```python
from build123d import *

# Parameters (mm, degrees)
F0_W     = 72
F0_H     = 24
F1_DEPTH = 27
F2_T     = -1
F3_R     = 3.25
F4_DEPTH = 25
F5_W     = 72
F5_H     = 27
F5_R     = 3.25
F6_DEPTH = 1
F8_DEPTH = 1
F9_R     = 0.8


# Not quite as in the source:
# - a feature names something its author has since deleted; it is built from what else it names


with BuildPart() as f1:
    # F0 (on Front) → F1 (new body)
    with BuildSketch(Plane.XZ):
        Rectangle(F0_W, F0_H)
    extrude(amount=F1_DEPTH)

    # F2
    f2_openings = [f1.faces().sort_by_distance(p)[0] for p in [
        (36, -13.5, 0),
    ]]
    offset(amount=F2_T, openings=f2_openings)

    # F3 (on face) → F4 (cut)
    with BuildSketch(Plane.XY.offset(12)):
        with Locations((-18.75, -13.5)):
            Circle(F3_R)
    extrude(amount=-F4_DEPTH, mode=Mode.SUBTRACT)

    # F5 (on face) → F6 (cut)
    with BuildSketch(Plane(origin=(0, 0, -12), x_dir=(1, 0, 0), z_dir=(0, 0, -1))):
        with Locations((0, 13.5)):
            Rectangle(F5_W, F5_H)
        with Locations((-18.75, 13.5)):
            Circle(F5_R, mode=Mode.SUBTRACT)
    extrude(amount=-F6_DEPTH, mode=Mode.SUBTRACT)

    # F9
    f9_edges = [f1.edges().sort_by_distance(p)[0] for p in [
        (-36, -27, 0.5),
        (-36, 0, 0.5),
    ]]
    fillet(f9_edges, radius=F9_R)


with BuildPart() as f8:
    # F7 (on face) → F8 (new body)
    with BuildSketch(Plane.XY.offset(12)):
        with BuildLine():
            Line((-36, -1), (-36, -27))
            Line((-36, -27), (36, -27))
            Line((36, -27), (36, -16.75))
            Line((36, -16.75), (-18.75, -16.75))
            ThreePointArc((-18.75, -16.75), (-22, -13.5), (-18.75, -10.25))
            Line((-18.75, -10.25), (36, -10.25))
            Line((36, -10.25), (36, -1))
            Line((36, -1), (-36, -1))
        make_face()
    extrude(amount=F8_DEPTH)


solid = f1.part
```
Build history of the part. All positions in model axes, mm. A direction names the side the tool comes from. Round coordinates to 2 decimals unless told otherwise and drop trailing zeros. Write each loop counter-clockwise with the first axis right and the second up, starting at its lowest first coordinate (ties: lowest second). Pieces come first, ordered by that corner, then holes.
1) Band-saw the part on B-B, the plane x = -18.75. List the corners of the cut face in (y, z).
2) Mould opens along Y. For faces 3 (the flat face through (0, 0, 1)), 4 (the flat face through (-36, -13, 0)), 5 (the cylindrical face through (-22, -13.4, 11.5)), 6 (the flat face through (0, -13, 11)) say: +Y half, -Y half, draft (parallel to the pull), parting line (faces both ways), or undercut.
3) Drill centre lines: probe 1 along Y at (x, z) = (-33, 5); probe 2 along Y at (x, z) = (-18.75, 11.6); probe 3 along Z at (x, y) = (31.5, -8.75). Where is each one in solid material? Low to high.
4) Band-saw the part on D-D, the plane z = -3. List the corners of the cut face in (x, y).
5) Pin check, flat tips, straight feed: pin 1 (1 mm diameter, centred on y = -5.5, z = 0, fed in from +X); pin 2 (2 mm diameter, centred on x = 12.5, y = -19.5, fed in from -Z). Stop position of each tip, or through.
6) Band-saw the part on A-A, the plane y = -13.5. List the corners of the cut face in (x, z), and give its area (3 significant figures).
7) Band-saw the part on C-C, the plane x = -26.5. List the corners of the cut face in (y, z).
8) 3-axis set-ups, long thin cutter, end or side, ignore diameter. For faces 1 (the flat face through (-0.2, -0.6, -11)), 2 (the flat face through (-35, -13, 0)): which of +Z, -Z, +X, -X, +Y, -Y reach the whole face in a straight line?
Ans:
1. outline: (-27, -11) - (-26, -11) - (-26, 11) - (-16.75, 11) - (-16.75, 12) - (-27, 12) - close; (-10.25, 11) - (-1, 11) - (-1, -11) - (0, -11) - (0, 12) - (-10.25, 12) - close
2. face 3: +Y half
2. face 4: draft
2. face 5: undercut
2. face 6: undercut
3. probe 1: y = -27 to -26, -1 to 0
3. probe 2: y = -27 to -16.75, -10.25 to 0
3. probe 3: z = 11 to 12
4. outline: (-36, -26.2) arc R0.8 ccw to (-35.2, -27) - (36, -27) - (36, -26) - (-35, -26) - (-35, -1) - (36, -1) - (36, 0) - (-35.2, 0) arc R0.8 ccw to (-36, -0.8) - close
5. pin 1: stops at x = -35
5. pin 2: stops at z = 11
6. outline: (-36, -11) - (-35, -11) - (-35, 11) - (-22, 11) - (-22, 12) - (-36, 12) - close; (-15.5, 11) - (36, 11) - (36, 12) - (-15.5, 12) - close
6. area: 87.5 mm2
7. outline: (-27, -11) - (-26, -11) - (-26, 11) - (-1, 11) - (-1, -11) - (0, -11) - (0, 12) - (-27, 12) - close
8. face 1: -Z, +X, -X, +Y, -Y
8. face 2: -Z, +X
